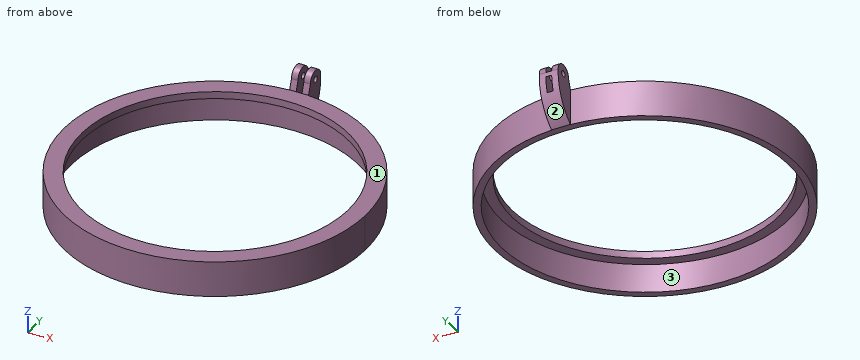
from build123d import *

# Parameters (mm, degrees)
SKETCH1_R                = 63.5
BOSS_EXTRUDE2_DEPTH      = 15
SHELL4_T                 = -3
SKETCH4_R                = 56.09702957
CUT_EXTRUDE1_DEPTH       = 22
BOSS_EXTRUDE6_DEPTH      = 4
BOSS_EXTRUDE6_DEPTH_BACK = 4
SKETCH8_R                = 1.3
BOSS_EXTRUDE7_REACH      = 145.843
BOSS_EXTRUDE7_END_RADIUS = 63.5
SKETCH9_W                = 8
SKETCH9_H                = 15
CUT_EXTRUDE2_DEPTH       = 9
CUT_EXTRUDE2_DEPTH_BACK  = 4
SKETCH10_W               = 2.5
SKETCH10_H               = 9.228481295


with BuildPart() as part:
    # Sketch1 → Boss-Extrude2 (new body)
    with BuildSketch(Plane.XY):
        Circle(SKETCH1_R)
    extrude(amount=BOSS_EXTRUDE2_DEPTH)

    # Shell4
    shell4_openings = [part.faces().sort_by_distance(p)[0] for p in [
        (0, 0, 0),
    ]]
    offset(amount=SHELL4_T, openings=shell4_openings, kind=Kind.INTERSECTION)

    # Sketch4 → Cut-Extrude1 (cut)
    with BuildSketch(Plane(origin=(0, 0, 12), x_dir=(-1, 0, 0), z_dir=(0, 0, -1))):
        Circle(SKETCH4_R)
    extrude(amount=-CUT_EXTRUDE1_DEPTH, mode=Mode.SUBTRACT)



with BuildPart() as body_2:
    # Sketch8 → Boss-Extrude6 (new, two sides: drawn at the far end of the back side and taken through both)
    with BuildSketch(Plane(origin=(0, 0, 0), x_dir=(0, 0, -1), z_dir=(1, 0, 0)).offset(-BOSS_EXTRUDE6_DEPTH_BACK)):
        with BuildLine():
            Line((-15, 63.5), (0, 63.5))
            ThreePointArc((0, 63.5), (-8.388517362, 70.509736152), (-19.092759253, 72.728481295))
            ThreePointArc((-19.092759253, 72.728481295), (-23.009560108, 68.811680441), (-19.092759253, 64.894879586))
            ThreePointArc((-19.092759253, 64.894879586), (-17.050704692, 64.184749485), (-15, 63.5))
        make_face()
        with Locations((-19.092759253, 68.811680441)):
            Circle(SKETCH8_R, mode=Mode.SUBTRACT)
    extrude(amount=BOSS_EXTRUDE6_DEPTH + BOSS_EXTRUDE6_DEPTH_BACK)


with BuildPart() as part_1:
    add(part.part)

    add(body_2.part)  # Boss-Extrude7 merges body 2
    # Boss-Extrude7: up to this cylinder (the profile starts outside it)
    boss_extrude7_end = Plane(origin=(0, 0, 7.5), z_dir=(0, 0, -1)) * Cylinder(BOSS_EXTRUDE7_END_RADIUS, 419.686, mode=Mode.PRIVATE)
    # Sketch9 → Boss-Extrude7 (add, up to the surface)
    with BuildSketch(Plane.XZ.offset(-63.5), mode=Mode.PRIVATE) as boss_extrude7_sk1:
        with Locations((0, 7.5)):
            Rectangle(SKETCH9_W, SKETCH9_H)
    boss_extrude7_tool1 = extrude(boss_extrude7_sk1.sketch, amount=BOSS_EXTRUDE7_REACH, mode=Mode.PRIVATE) - boss_extrude7_end
    add(boss_extrude7_tool1.solids().sort_by_distance((0, 63.5, 7.5))[0])
    add(boss_extrude7_tool1.solids().sort_by_distance((0, 63.5, 7.5))[1])

    # Sketch10 → Cut-Extrude2 (cut, two sides: drawn at the far end of the back side and taken through both)
    with BuildSketch(Plane.XY.offset(15).offset(-CUT_EXTRUDE2_DEPTH_BACK)):
        with Locations((0, 68.114240648)):
            Rectangle(SKETCH10_W, SKETCH10_H)
    extrude(amount=CUT_EXTRUDE2_DEPTH + CUT_EXTRUDE2_DEPTH_BACK, mode=Mode.SUBTRACT)


solid = part_1.part
Input: part model. Units: mm. Frame: model coordinates. Face numbers are marked on the shaded views. Give positions to 0.01 mm unless a question says otherwise; leave off trailing zeros. Loops run counter-clockwise (first coordinate to the right, second up) from the corner with the lowest first, then second, coordinate; pieces in that order, holes last. Notation, with made-up numbers: (-19, 20.5) -> (-13, 20.5) arc R36 cw to (-13, 55.5) -> close; hole circle Ø1 at (24.25, 47.25). An arc over 180 degrees is marked (long way). Answer as a JSON object with one key per item and string values. Group by question number.
Item 1: Cut plane A-A, the plane y = -49. Return the cut outline in (x, z), and give its area (3 significant figures).
Item 2: Pull-direction query (Y, two-part tool) for the marked faces 1, 2 and 3; classes: released by +Y, released by -Y, zero draft, split by the parting line, or undercut.
Item 3: Cut plane C-C, the plane z = 2.25. Return the cut outline in (x, y).
Item 4: Cut plane B-B, the plane x = -20.5. Return the cut outline in (y, z), and give its area (3 significant figures).
Item 5: Pin query (flat end, axial travel): P1, Ø2, axis at x = 13, z = 5.5, coming from the +Y side; P2, Ø1.2, axis at x = 0.5, y = 66, coming from the +Z side; P3, Ø1.5, axis at y = 35, z = 5.5, coming from the +X side. Return the tip coordinate at first contact, or that it passes through.
Item 6: Cut plane D-D, the plane z = 9. Return the cut outline in (x, y), and give its area (3 significant figures).
Item 7: Line query: probe 1 along Y at (x, z) = (0, 12.6); probe 2 along X at (y, z) = (0, 8.25); probe 3 along X at (y, z) = (12.5, 11). Output: solid intervals per line, ascending.
Checks:
{
 "1": {"outline": "(-40.39, 0) -> (-35.49, 0) -> (-35.49, 12) -> (-27.31, 12) -> (-27.31, 15) -> (-40.39, 15) -> close; (27.31, 12) -> (35.49, 12) -> (35.49, 0) -> (40.39, 0) -> (40.39, 15) -> (27.31, 15) -> close", "area": "196 mm²"},
 "2": {"face 1": "zero draft", "face 2": "released by +Y", "face 3": "undercut"},
 "3": {"outline": "(-4, 63.37) arc R63.5 ccw (long way) to (4, 63.37) -> (4, 66.14) -> (-4, 66.14) -> close; hole circle Ø121 at (0, 0)"},
 "4": {"outline": "(-60.1, 0) -> (-56.92, 0) -> (-56.92, 12) -> (-52.22, 12) -> (-52.22, 15) -> (-60.1, 15) -> close; (52.22, 12) -> (56.92, 12) -> (56.92, 0) -> (60.1, 0) -> (60.1, 15) -> (52.22, 15) -> close", "area": "124 mm²"},
 "5": {"P1": "stops at y = 62.36", "P2": "stops at z = 11", "P3": "stops at x = 53.47"},
 "6": {"outline": "(-4, 63.37) arc R63.5 ccw (long way) to (4, 63.37) -> (4, 70.79) -> (-4, 70.79) -> close; hole circle Ø121 at (0, 0)", "area": "1,230 mm²"},
 "7": {"probe 1": "y = -63.5 to -56.1, 56.1 to 63.5", "probe 2": "x = -63.5 to -60.5, 60.5 to 63.5", "probe 3": "x = -62.26 to -59.19, 59.19 to 62.26"}
}
